Part model, mm, in its own coordinate system. A direction names the side the tool comes from. Give positions to 0.01 mm unless a question says otherwise; leave off trailing zeros. Loops run counter-clockwise (first coordinate to the right, second up) from the corner with the lowest first, then second, coordinate; pieces in that order, holes last. Notation, with made-up numbers: M -7,70 L 49,70 A12 ccw 49,75 Z; hole C 21.5,75.25 d11. An arc over 180 degrees is marked long. Put each result on its own line as item: value. Start each with the question number.
```python
from build123d import *

# Parameters (mm, degrees)
SKETCH1_R            = 1.54
BOSS_EXTRUDE1_DEPTH  = 1
SKETCH2_W            = 15
SKETCH2_H            = 15
BOSS_EXTRUDE2_DEPTH  = 2
SKETCH3_W            = 10
SKETCH3_H            = 15
BOSS_EXTRUDE3_DEPTH  = 2
SKETCH4_W            = 50.8
SKETCH4_H            = 5.26
SKETCH4_H_2          = 4.9
BOSS_EXTRUDE4_DEPTH  = 9.2
SKETCH5_W            = 14.5
SKETCH5_H            = 12
BOSS_EXTRUDE6_DEPTH  = 7
SKETCH6_W            = 12
SKETCH6_H            = 5
BOSS_EXTRUDE7_DEPTH  = 5
SKETCH7_R            = 2.25
BOSS_EXTRUDE8_DEPTH  = 2
SKETCH8_W            = 6
SKETCH8_H            = 6.92
BOSS_EXTRUDE9_DEPTH  = 4
SKETCH9_W            = 6
SKETCH9_H            = 5
BOSS_EXTRUDE10_DEPTH = 4
SKETCH10_W           = 12
SKETCH10_H           = 18.48
BOSS_EXTRUDE11_DEPTH = 1
SKETCH11_W           = 12
SKETCH11_H           = 12
BOSS_EXTRUDE12_DEPTH = 1
SKETCH12_W           = 4
SKETCH12_H           = 4
BOSS_EXTRUDE13_DEPTH = 1
SKETCH13_W           = 2
SKETCH13_H           = 5
BOSS_EXTRUDE14_DEPTH = 0.5
SKETCH14_R           = 0.75
BOSS_EXTRUDE15_DEPTH = 0.5


with BuildPart() as part:
    # Sketch1 → Boss-Extrude1 (new body)
    with BuildSketch(Plane.XY):
        Polygon((0, 0), (-56.7, 0), (-60.5, -3.8), (-60.5, -41), (0, -41), align=None)
        with Locations((-56.5, -4)):
            Circle(SKETCH1_R, mode=Mode.SUBTRACT)
    extrude(amount=BOSS_EXTRUDE1_DEPTH)

    # Sketch2 → Boss-Extrude2 (add)
    with BuildSketch(Plane(origin=(0, 0, 0), x_dir=(-1, 0, 0), z_dir=(0, 0, -1))):
        with Locations((22.5, -14.5)):
            Rectangle(SKETCH2_W, SKETCH2_H)
    extrude(amount=-BOSS_EXTRUDE2_DEPTH)

    # Sketch3 → Boss-Extrude3 (add)
    with BuildSketch(Plane(origin=(0, 0, 0), x_dir=(-1, 0, 0), z_dir=(0, 0, -1))):
        with Locations((40.5, -26.5)):
            Rectangle(SKETCH3_W, SKETCH3_H)
    extrude(amount=-BOSS_EXTRUDE3_DEPTH)

    # Sketch4 → Boss-Extrude4 (add)
    with BuildSketch(Plane(origin=(0, 0, 0), x_dir=(-1, 0, 0), z_dir=(0, 0, -1))):
        with Locations((25.58, -38.19)):
            Rectangle(SKETCH4_W, SKETCH4_H)
        with Locations((25.58, -2.63)):
            Rectangle(SKETCH4_W, SKETCH4_H_2)
    extrude(amount=BOSS_EXTRUDE4_DEPTH)

    # Sketch5 → Boss-Extrude6 (add)
    with BuildSketch(Plane(origin=(0, 0, 0), x_dir=(-1, 0, 0), z_dir=(0, 0, -1))):
        with Locations((52.75, -14.08)):
            Rectangle(SKETCH5_W, SKETCH5_H)
    extrude(amount=BOSS_EXTRUDE6_DEPTH)

    # Sketch6 → Boss-Extrude7 (add)
    with BuildSketch(Plane(origin=(0, 0, 0), x_dir=(-1, 0, 0), z_dir=(0, 0, -1))):
        with Locations((51.5, -25.58)):
            Rectangle(SKETCH6_W, SKETCH6_H)
    extrude(amount=BOSS_EXTRUDE7_DEPTH)

    # Sketch7 → Boss-Extrude8 (add)
    with BuildSketch(Plane.ZY.offset(57.5)):
        with Locations(Location((-2.5, -25.58, 0), (0, 0, 180))):
            Circle(SKETCH7_R)
    extrude(amount=BOSS_EXTRUDE8_DEPTH)

    # Sketch8 → Boss-Extrude9 (add)
    with BuildSketch(Plane(origin=(0, 0, 0), x_dir=(-1, 0, 0), z_dir=(0, 0, -1))):
        with Locations((57, -36.54)):
            Rectangle(SKETCH8_W, SKETCH8_H)
    extrude(amount=BOSS_EXTRUDE9_DEPTH)

    # Sketch9 → Boss-Extrude10 (add)
    with BuildSketch(Plane(origin=(0, 0, 0), x_dir=(-1, 0, 0), z_dir=(0, 0, -1))):
        with Locations((3.5, -32.06)):
            Rectangle(SKETCH9_W, SKETCH9_H)
    extrude(amount=BOSS_EXTRUDE10_DEPTH)

    # Sketch10 → Boss-Extrude11 (add)
    with BuildSketch(Plane(origin=(0, 0, 0), x_dir=(-1, 0, 0), z_dir=(0, 0, -1))):
        with Locations((26, -19.32)):
            Rectangle(SKETCH10_W, SKETCH10_H)
    extrude(amount=BOSS_EXTRUDE11_DEPTH)

    # Sketch11 → Boss-Extrude12 (add)
    with BuildSketch(Plane(origin=(0, 0, 0), x_dir=(-1, 0, 0), z_dir=(0, 0, -1))):
        with Locations((10, -12.08)):
            Rectangle(SKETCH11_W, SKETCH11_H)
    extrude(amount=BOSS_EXTRUDE12_DEPTH)

    # Sketch12 → Boss-Extrude13 (add)
    with BuildSketch(Plane(origin=(0, 0, -1), x_dir=(-1, 0, 0), z_dir=(0, 0, -1))):
        with Locations((10, -11.08)):
            Rectangle(SKETCH12_W, SKETCH12_H)
    extrude(amount=BOSS_EXTRUDE13_DEPTH)

    # Sketch13 → Boss-Extrude14 (add)
    with BuildSketch(Plane(origin=(0, 0, 0), x_dir=(-1, 0, 0), z_dir=(0, 0, -1))):
        with Locations((2, -8.58)):
            Rectangle(SKETCH13_W, SKETCH13_H)
    extrude(amount=BOSS_EXTRUDE14_DEPTH)

    # Sketch14 → Boss-Extrude15 (add)
    with BuildSketch(Plane(origin=(0, 0, -0.5), x_dir=(-1, 0, 0), z_dir=(0, 0, -1))):
        with Locations(Location((2.037351084, -8.580279036, 0), (0, 0, 180))):
            Circle(SKETCH14_R)
    extrude(amount=BOSS_EXTRUDE15_DEPTH)


solid = part.part
```
1) Mould opens along Z. For faces 1 (the flat face through (-0.18, -38, -5)), 2 (the flat face through (-2, -9, -1)), 3 (the flat face through (-57.5, -27.3, -0.8)) say: +Z half, -Z half, draft (parallel to the pull), parting line (faces both ways), or undercut.
2) Pin check, flat tips, straight feed: pin 1 Ø5 at (x, z) = (-36, -4.5) entering from +Y; pin 2 Ø1.5 at (x, z) = (-41.5, -7.5) entering from -Y; pin 3 Ø0.8 at (y, z) = (-15, -0.5) entering from -X; pin 4 Ø1.8 at (x, y) = (-56.5, -4) entering from -Z. Stop position of each tip, or through.
3) Which spindle directions (+Z, -Z, +X, -X, +Y, -Y) get a long thin tool onto all of the face, cutting with end or side? Do faces 4 (the flat face through (-51, -23.08, -2)), 5 (the flat face through (-57, -40, -2)), 6 (the flat face through (-45.5, -14, -3)), 7 (the flat face through (-10, -11, -2)). Say none if no direction does.
4) Band-saw the part on B-B on x = -28.5. Give the cut face in (y, z), then the cut area to 3 significant figures.
5) Band-saw the part on A-A on y = -25.58. Give the cut face in (x, z), then the cut area to 4 significant figures.
6) Band-saw the part on D-D on x = -44. Give the cut face in (y, z).
7) Wall check: L1, parallel to Y at x = -49, z = -6.5; L2, parallel to Y at x = -56.5, z = 0.5; L3, parallel to Y at x = -23.5, z = -1.25. Give the ranges that are in metal, low to high.
8) Band-saw the part on C-C on x = -13. Give the cut face in (y, z).
Evaluation:
1. face 1: draft
1. face 2: -Z half
1. face 3: undercut
2. pin 1: y = -0.18
2. pin 2: y = -40.82
2. pin 3: x = -60
2. pin 4: through
3. face 4: -Z, -X
3. face 5: -Z, -X, -Y
3. face 6: -Z
3. face 7: -Z, +X
4. outline: M -41,0 L -40.82,0 L -40.82,-9.2 L -35.56,-9.2 L -35.56,0 L -28.56,0 L -28.56,-1 L -10.08,-1 L -10.08,0 L -5.08,0 L -5.08,-9.2 L -0.18,-9.2 L -0.18,0 L 0,0 L 0,1 L -7,1 L -7,2 L -22,2 L -22,1 L -41,1 Z
4. area: 168 mm2
5. outline: M -60.5,0 L -57.5,0 L -57.5,-0.25 L -59.5,-0.25 L -59.5,-4.75 L -57.5,-4.75 L -57.5,-5 L -45.5,-5 L -45.5,0 L -32,0 L -32,-1 L -20,-1 L -20,0 L 0,0 L 0,1 L -35.5,1 L -35.5,2 L -45.5,2 L -45.5,1 L -60.5,1 Z
5. area: 151.5 mm2
6. outline: M -41,0 L -40.82,0 L -40.82,-9.2 L -35.56,-9.2 L -35.56,0 L -5.08,0 L -5.08,-9.2 L -0.18,-9.2 L -0.18,0 L 0,0 L 0,1 L -19,1 L -19,2 L -34,2 L -34,1 L -41,1 Z
7. L1: -40.82 to -35.56, -20.08 to -8.08, -5.08 to -0.18
7. L2: -41 to -5.54, -2.46 to 0
7. L3: -40.82 to -35.56, -5.08 to -0.18
8. outline: M -41,0 L -40.82,0 L -40.82,-9.2 L -35.56,-9.2 L -35.56,0 L -18.08,0 L -18.08,-1 L -6.08,-1 L -6.08,0 L -5.08,0 L -5.08,-9.2 L -0.18,-9.2 L -0.18,0 L 0,0 L 0,1 L -41,1 Z
